Could you check a few things on this model? Use its own coordinates, in mm. A direction names the side the tool comes from. Round coordinates to 2 decimals unless told otherwise and drop trailing zeros. Write each loop counter-clockwise with the first axis right and the second up, starting at its lowest first coordinate (ties: lowest second). Pieces come first, ordered by that corner, then holes. Notation, with made-up numbers: (-5, 1.25) -> (45, 1.25) arc R18 cw to (45, 34.25) -> close; hole circle Ø3 at (49, 38.5). An arc over 180 degrees is marked (long way). Answer as CSV lines item,"result". Start each with the question number.
Q1. Imagine slicing it at C-C on y = 14.25. Please give me the cut outline in (x, z), and give its area (3 significant figures).
Q2. If I drill on line 1 (X direction, y = 11.15, z = 0); line 2 (Y direction, x = -10.8, z = 0); line 3 (X direction, y = 8.35, z = 0), over which ranges is the centre line in solid material (lowest first)? Write a range as [from, to].
Q3. For faces 5 (the cylindrical face through (-10.93, 3.31, -1.55)), 6 (the flat face through (-10, 7, 3)), 7 (the flat face through (-5, 11.5, 0)), 8 (the flat face through (4, 19.5, -2)), which set-ups out of +Z, -Z, +X, -X, +Y, -Y let a thin tool reach every point of the face, with its end or its side?
Q4. Imagine slicing it at D-D on z = 3.25. Please give me the cut outline in (x, y).
Q5. Imagine slicing it at A-A on z = 0. Please give me the cut outline in (x, y), and give its area (3 significant figures).
Q6. Imagine slicing it at B-B on x = -0.5. Please give me the cut outline in (y, z).
Q7. If we mould it in two halves opening along X, with no side actions, what happens to faces 1 (the cylindrical face through (0.08, 11.01, -1.9)), 2 (the flat face through (-1, 0, 11)), 3 (the cylindrical face through (-4.59, 15.44, -1.02)), 4 (the cylindrical face through (10.66, 3.55, -1.4))? For each: pulls with the +X half, pulls with the -X half, needs draft (parallel to the pull), parting line crosses it, or undercut.
Q8. Will these pins go through, and if not, where does the flat tip stop? pin 1 Ø8 at (x, z) = (5, -0.5) entering from -Y; pin 2 Ø1 at (x, z) = (9, 3) entering from +Y; pin 3 Ø3 at (y, z) = (2.5, 0) entering from -X.
from build123d import *

# Parameters (mm, degrees)
F2_R     = 1.75
F3_DEPTH = 11.251


with BuildPart() as f1:
    # F0 (on Right) → F1 (revolve)
    with BuildSketch(Plane.YZ):
        Polygon((11.5, 11.25), (0, 11.25), (0, 10.75), (7, 10.75), (7, 10), (10.5, 10), (10.5, 1.9), (11.5, 1.9), (11.5, 4), (19.5, 4), (19.5, 4.7), (11.5, 4.7), align=None)
    revolve(axis=Axis((0, 13.454885, 0), (0, 1, 0)))

    # F2 (on Right) → F3 (cut, through all)
    with BuildSketch(Plane.YZ):
        with Locations((2.5, 0)):
            Circle(F2_R)
    extrude(amount=-F3_DEPTH, mode=Mode.SUBTRACT)


solid = f1.part
Checks:
1,outline,"circle Ø9.4 at (0, 0); hole circle Ø8 at (0, 0)"
1,area,"19.1 mm^2"
2,line 1,"[-11.25, -1.9], [1.9, 11.25]"
2,line 2,"[0, 0.75], [4.25, 11.5]"
2,line 3,"[-11.25, -10], [10, 11.25]"
3,face 5,"-X"
3,face 6,"-Y"
3,face 7,"+Y"
3,face 8,"+Z, -Z, +X, -X, +Y"
4,outline,"(-10.77, 0) -> (-10.25, 0) -> (-10.25, 7) -> (-9.46, 7) -> (-9.46, 10.5) -> (9.46, 10.5) -> (9.46, 7) -> (10.25, 7) -> (10.25, 0) -> (10.77, 0) -> (10.77, 11.5) -> (3.4, 11.5) -> (3.4, 19.5) -> (2.33, 19.5) -> (2.33, 11.5) -> (-2.33, 11.5) -> (-2.33, 19.5) -> (-3.4, 19.5) -> (-3.4, 11.5) -> (-10.77, 11.5) -> close"
5,outline,"(-11.25, 0) -> (-10.75, 0) -> (-10.75, 0.75) -> (-11.25, 0.75) -> close; (-11.25, 4.25) -> (-10.75, 4.25) -> (-10.75, 7) -> (-10, 7) -> (-10, 10.5) -> (-1.9, 10.5) -> (-1.9, 11.5) -> (-4, 11.5) -> (-4, 19.5) -> (-4.7, 19.5) -> (-4.7, 11.5) -> (-11.25, 11.5) -> close; (1.9, 10.5) -> (10, 10.5) -> (10, 7) -> (10.75, 7) -> (10.75, 0) -> (11.25, 0) -> (11.25, 11.5) -> (4.7, 11.5) -> (4.7, 19.5) -> (4, 19.5) -> (4, 11.5) -> (1.9, 11.5) -> close"
5,area,"43.9 mm^2"
6,outline,"(0, -11.24) -> (11.5, -11.24) -> (11.5, -4.67) -> (19.5, -4.67) -> (19.5, -3.97) -> (11.5, -3.97) -> (11.5, -1.83) -> (10.5, -1.83) -> (10.5, -9.99) -> (7, -9.99) -> (7, -10.74) -> (0, -10.74) -> close; (0, 10.74) -> (7, 10.74) -> (7, 9.99) -> (10.5, 9.99) -> (10.5, 1.83) -> (11.5, 1.83) -> (11.5, 3.97) -> (19.5, 3.97) -> (19.5, 4.67) -> (11.5, 4.67) -> (11.5, 11.24) -> (0, 11.24) -> close"
7,face 1,"undercut"
7,face 2,"needs draft"
7,face 3,"parting line crosses it"
7,face 4,"undercut"
8,pin 1,"y = 10.5"
8,pin 2,"y = 11.5"
8,pin 3,"x = 10.64"
